The model under review builds one solid part; all positions refer to its coordinate system, in mm. Face numbers are marked on the shaded views. A direction names the side the tool comes from. Coordinates: 2 decimals unless noted, no trailing zeros. Write each loop counter-clockwise with the first axis right and the second up, starting at its lowest first coordinate (ties: lowest second). Pieces come first, ordered by that corner, then holes. Notation, with made-up numbers: M 57.25,-26.5 L 100.25,-26.5 A18 cw 100.25,-1.5 Z; hole C 49,80 d2. An arc over 180 degrees is marked long. Answer as a JSON object with one key per item and string values.
Autodesk Inventor part; units mm, degrees
ref_plane "YZ Plane" through (0, 0, 0) normal (1, 0, 0) x (0, 1, 0)
ref_plane "XZ Plane" through (0, 0, 0) normal (0, 1, 0) x (-1, 0, 0)
ref_plane "XY Plane" through (0, 0, 0) normal (0, 0, 1) x (1, 0, 0)
sketch "草图1" plane through (0, 0, 0) normal (0, 1, 0) x (-1, 0, 0)
  line L0 (68.3073, 0) -> (21.1081, -64.9641)
  line L1 (21.1081, -64.9641) -> (-55.2617, -40.15)
  line L2 (-55.2617, -40.15) -> (-55.2617, 40.15)
  line L3 (-55.2617, 40.15) -> (21.1081, 64.9641)
  line L4 (21.1081, 64.9641) -> (68.3073, 0)
  line L5 (105.0554, 0) -> (32.4639, -99.9136)
  line L6 (32.4639, -99.9136) -> (-84.9916, -61.75)
  line L7 (-84.9916, -61.75) -> (-84.9916, 61.75)
  line L8 (-84.9916, 61.75) -> (32.4639, 99.9136)
  line L9 (32.4639, 99.9136) -> (105.0554, 0)
  point P0 (0, 0)
  point P1 (0, 0)
  point P2 (0, 0)
  dimension "d0" = 80.3
  dimension "d1" = 123.5
extrude "拉伸1" add sketch "草图1" along normal blind 2
sketch "草图2" plane through (0, 2, 0) normal (0, 1, 0) x (1, 0, 0)
  line L0 (-21.1081, 64.9641) -> (55.2617, 40.15)
  line L1 (55.2617, 40.15) -> (55.2617, -40.15)
  line L2 (55.2617, -40.15) -> (-21.1081, -64.9641)
  line L3 (-21.1081, -64.9641) -> (-68.3073, 0)
  line L4 (-68.3073, 0) -> (-21.1081, 64.9641)
  line L5 (-32.4639, 99.9136) -> (-105.0554, 0)
  line L6 (-105.0554, 0) -> (-32.4639, -99.9136)
  line L7 (-32.4639, -99.9136) -> (84.9916, -61.75)
  line L8 (84.9916, -61.75) -> (84.9916, 61.75)
  line L9 (84.9916, 61.75) -> (-32.4639, 99.9136)
  line L10 (58.7617, 42.6929) -> (-22.445, 69.0786)
  line L11 (-22.445, 69.0786) -> (-72.6335, 0)
  line L12 (-72.6335, 0) -> (-22.445, -69.0786)
  line L13 (-22.445, -69.0786) -> (58.7617, -42.6929)
  line L14 (58.7617, -42.6929) -> (58.7617, 42.6929)
  line L15 (-23.2089, 71.4297) -> (60.7617, 44.146)
  line L16 (60.7617, 44.146) -> (60.7617, -44.146)
  line L17 (60.7617, -44.146) -> (-23.2089, -71.4297)
  line L18 (-23.2089, -71.4297) -> (-75.1056, 0)
  line L19 (-75.1056, 0) -> (-23.2089, 71.4297)
  point P0 (0, 0)
  dimension "d4" = 3.5
  dimension "d5" = 2
extrude "拉伸2" add sketch "草图2" along normal blind 10 contours L15 L16 L17 L18 L19
sketch "草图3" plane through (0, 0, 0) normal (0, -1, 0) x (1, 0, 0)
  line L0 (-9.4145, -72.1274) -> (53.3776, -50.8644)
  line L1 (53.3776, -50.8644) -> (57.7542, -63.7889)
  line L2 (57.7542, -63.7889) -> (-5.038, -85.0518)
  line L3 (-5.038, -85.0518) -> (-9.4145, -72.1274)
  point P0 (0, 0)
extrude "拉伸3" cut sketch "草图3" against normal blind 10
sketch "草图4" plane through (0, 0, 0) normal (0, -1, 0) x (1, 0, 0)
  line L0 (-105.0554, 0) -> (-32.4639, -99.9136)
  line L1 (-105.0554, 0) -> (0, 0)
  line L2 (0, 0) -> (99.3977, 72.2167)
  line L3 (99.3977, 72.2167) -> (-62.0091, 125.592)
  line L4 (-62.0091, 125.592) -> (-127.7953, 9.1282)
  line L5 (-127.7953, 9.1282) -> (-105.0554, 0)
extrude "拉伸4" cut sketch "草图4" against normal blind 20
properties part number "上部端盖" material "橡胶"
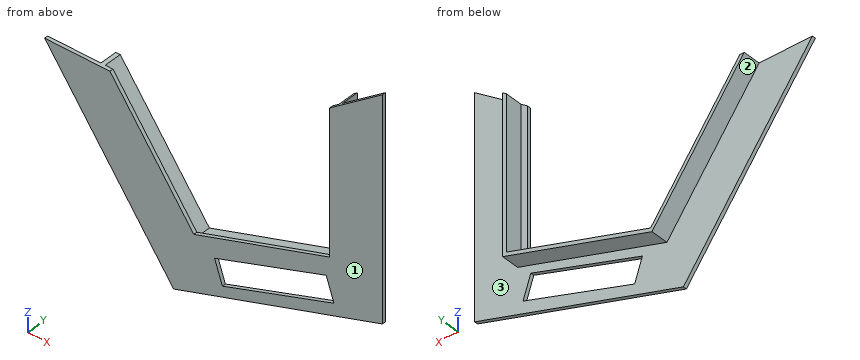
(1) Add section D-D on y = 7.5. Give the boundary of the cut face in (x, z) (1 decimal).
Results list:
{"outline": "M -75.1,0 L -23.2,-71.4 L 60.8,-44.1 L 60.8,44.1 L 58.8,42.7 L 58.8,-42.7 L -22.4,-69.1 L -72.6,0 Z"}
(2) Wall thickness on line 1 along X through (y, z) = (7, 14.5); line 2 along Y through (x, z) = (-32, -67); line 3 along X through (y, z) = (7.5, -23): over which ranges is each line inside the solid? List them lowest first. Write a range as from..to.
Results list:
{"line 1": "58.76..60.76", "line 2": "0..2", "line 3": "-58.4..-55.92, 58.76..60.76"}
(3) For the marked faces 1, 2 and 3, list the 3-axis set-ups (+Z, -Z, +X, -X, +Y, -Y) from which the entire face can be reached by the end or side of a thin tool; tool diameter is ignored.
Results list:
{"face 1": "+Z, -Z, +X, -X, -Y", "face 2": "-Z, -X, +Y", "face 3": "-Z, +Y"}
(4) Add section A-A on z = 24. Give the boundary of the cut face in (x, y), and give its area (3 significant figures).
Results list:
{"outline": "M 55.26,0 L 84.99,0 L 84.99,2 L 60.76,2 L 60.76,12 L 58.76,12 L 58.76,2 L 55.26,2 Z", "area": "79.5 mm²"}
(5) Add section B-B on z = -14.5. Give the boundary of the cut face in (x, y).
Results list:
{"outline": "M -94.52,0 L -57.77,0 L -57.77,2 L -62.1,2 L -62.1,12 L -64.57,12 L -64.57,2 L -94.52,2 Z; M 55.26,0 L 84.99,0 L 84.99,2 L 60.76,2 L 60.76,12 L 58.76,12 L 58.76,2 L 55.26,2 Z"}
(6) For pin 1 Ø1.6 at (y, z) = (1, -9.5) entering from -X; pin 2 Ø4 at (y, z) = (1.5, 5) entering from -X; pin 3 Ø4 at (x, y) = (1, 5.5) entering from -Z, all flat-tipped, find the tip position at first contact; note any pin that passes through.
Results list:
{"pin 1": "x = -98.73", "pin 2": "x = 55.26", "pin 3": "z = -64.21"}
(7) Add section C-C on x = 18.5. Give the boundary of the cut face in (y, z), and give its area (3 significant figures).
Results list:
{"outline": "M 0,-83.35 L 2,-83.35 L 2,-77.08 L 0,-77.08 Z; M 0,-62.67 L 2,-62.67 L 2,-57.88 L 12,-57.88 L 12,-55.77 L 2,-55.77 L 2,-52.09 L 0,-52.09 Z", "area": "54.7 mm²"}
